Work out the finished part from the listing and answer in its coordinate system (mm). Face numbers are marked on the shaded views. Round coordinates to 2 decimals unless told otherwise and drop trailing zeros. Loops run counter-clockwise (first coordinate to the right, second up) from the corner with the lowest first, then second, coordinate; pieces in that order, holes last.
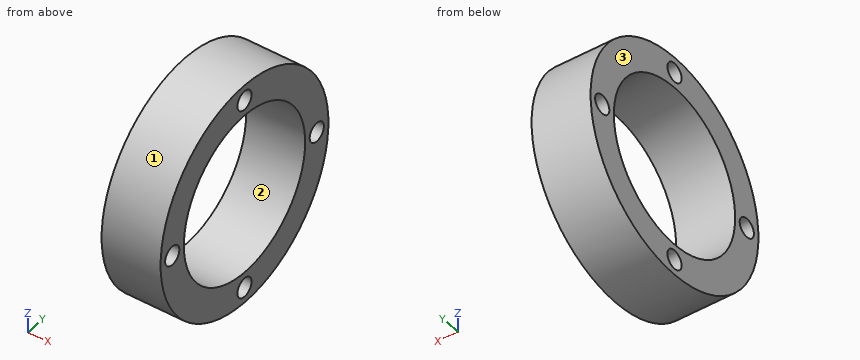
```python
from build123d import *

# Parameters (mm, degrees)
F0_W = 17
F0_H = 9
F3_D = 5.5


with BuildPart() as f1:
    # F0 (on Front) → F1 (revolve)
    with BuildSketch(Plane.XZ):
        with Locations((8.5, 28)):
            Rectangle(F0_W, F0_H)
    revolve(axis=Axis((1.6395361068, 0, 0), (1, 0, 0)))

    # F3 (through all)
    with Locations(Plane(origin=(0, 0, 0), x_dir=(0, -1, 0), z_dir=(-1, 0, 0))):
        with Locations((0, 28), (28, 0), (0, -28), (-28, 0)):
            Hole(F3_D / 2)


solid = f1.part
```
1. Find section A-A (z = 0). Write down the section's boundary in (x, y).
Answer key:
outline: (0, -32.5) - (17, -32.5) - (17, -30.75) - (0, -30.75) - close; (0, -25.25) - (17, -25.25) - (17, -23.5) - (0, -23.5) - close; (0, 23.5) - (17, 23.5) - (17, 25.25) - (0, 25.25) - close; (0, 30.75) - (17, 30.75) - (17, 32.5) - (0, 32.5) - close
2. Consider probe 1 along Z at (x, y) = (8.75, 0); probe 2 along Y at (x, z) = (2.75, 8). Determine where each line is inside the solid, lowest interval first.
Answer key:
probe 1: z = -32.5 to -30.75, -25.25 to -23.5, 23.5 to 25.25, 30.75 to 32.5
probe 2: y = -31.5 to -22.1, 22.1 to 31.5
3. Find section D-D (x = 10). Write down the section's boundary in (y, z), then the cut area to 3 significant figures.
Answer key:
outline: circle Ø65 at (0, 0); hole circle Ø5.5 at (-28, 0); hole circle Ø47 at (0, 0); hole circle Ø5.5 at (0, -28); hole circle Ø5.5 at (0, 28); hole circle Ø5.5 at (28, 0)
area: 1,490 mm2
4. Find section C-C (z = -28). Write down the section's boundary in (x, y).
Answer key:
outline: (0, -16.5) - (17, -16.5) - (17, -2.75) - (0, -2.75) - close; (0, 2.75) - (17, 2.75) - (17, 16.5) - (0, 16.5) - close
5. Given pin 1 (5 mm diameter, centred on x = 6.5, y = -23, fed in from -Z); pin 2 (10 mm diameter, centred on x = 14, z = 14.5, fed in from +Y); pin 3 (6 mm diameter, centred on x = 4.5, y = 17.5, fed in from -Z); pin 4 (4.5 mm diameter, centred on y = 0, z = 28, fed in from -X), each flat-ended and moving along its own axis, determine where each tip first touches the part or whether it passes through.
Answer key:
pin 1: stops at z = -25.22
pin 2: stops at y = 31.08
pin 3: stops at z = -29.09
pin 4: passes through
6. Determine the mould class of the marked faces 1, 2 and 3 for opening direction Z: +Z half, -Z half, draft (parallel to the pull), parting line (faces both ways), or undercut.
Answer key:
face 1: parting line
face 2: undercut
face 3: draft
